Could you check a few things on this drawing? It's one solid part, dimensions in mm from its lowest x, y, z. A direction names the side the tool comes from. Give positions to 0.01 mm unless a question says otherwise; leave off trailing zeros. Loops run counter-clockwise (first coordinate to the right, second up) from the corner with the lowest first, then second, coordinate; pieces in that order, holes last. Notation, with made-up numbers: (-29.75, 31.25) -> (-2.75, 31.25) arc R7 cw to (-2.75, 39.25) -> close; hole circle Ø5 at (39, 38). An arc over 180 degrees is marked (long way). One line per question, with ' | ' between items.
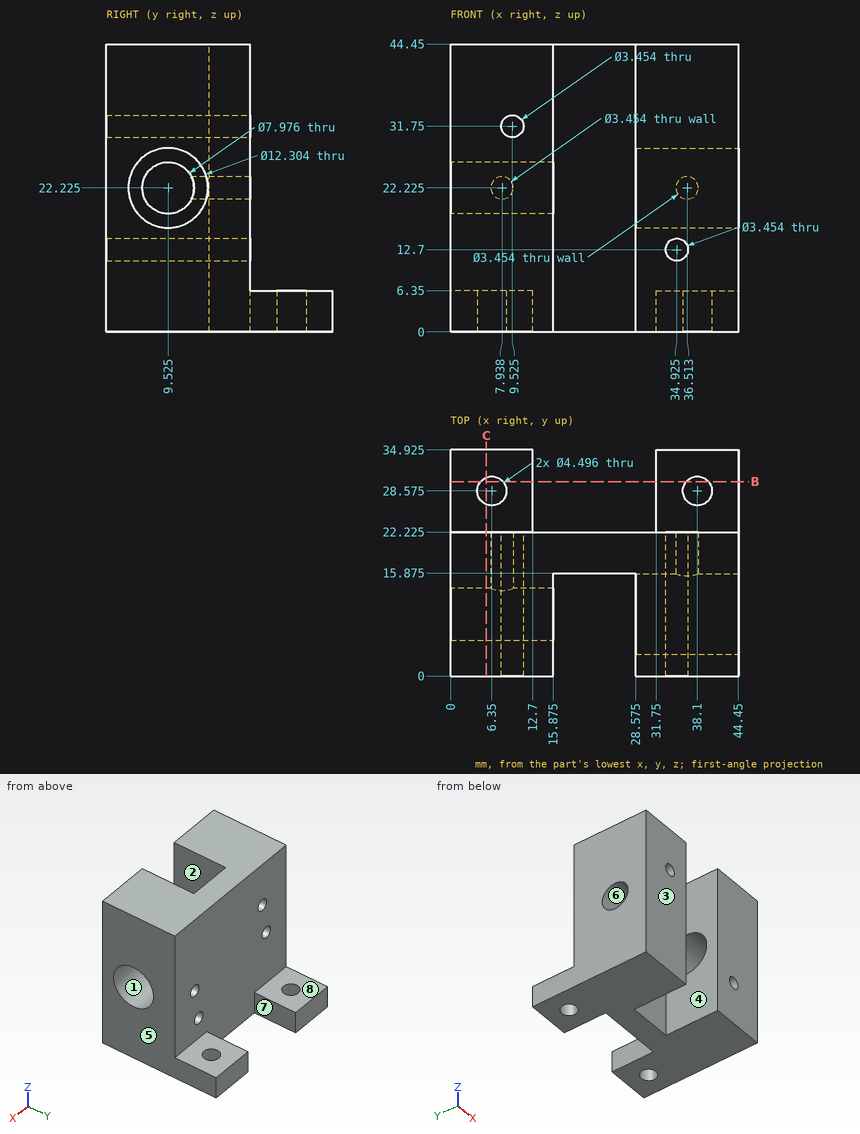
Q1. If we section it at B-B (y = 30): Write out the boundary of the cut face in (x, z).
Entries:
outline: (0, 0) -> (4.61, 0) -> (4.61, 6.35) -> (0, 6.35) -> close; (8.09, 0) -> (12.7, 0) -> (12.7, 6.35) -> (8.09, 6.35) -> close; (31.75, 0) -> (36.36, 0) -> (36.36, 6.35) -> (31.75, 6.35) -> close; (39.84, 0) -> (44.45, 0) -> (44.45, 6.35) -> (39.84, 6.35) -> close
Q2. If we mould it in two halves opening along Y, with no side actions, what happens to the marked faces 1, 2 and 3? For each: pulls with the +Y half, pulls with the -Y half, needs draft (parallel to the pull), parting line crosses it, or undercut.
Entries:
face 1: undercut | face 2: needs draft | face 3: pulls with the -Y half
Q3. If I drill on probe 1 along Y at (x, z) = (4, 41.5) (1 decimal); probe 2 along Z at (x, y) = (42, 31.5); probe 3 along Z at (x, y) = (38, 13.5), over which ranges is the centre line in solid material (lowest first)? Write a range as from..to.
Entries:
probe 1: 0..22.2 | probe 2: 0..6.35 | probe 3: 0..17.53, 26.92..44.45
Q4. For pin 1 Ø4 at (x, z) = (20.5, 6.5) entering from +Y (1 decimal); pin 2 Ø17.5 at (y, z) = (8.5, 24.5) entering from +X; pin 3 Ø5 at (x, y) = (34, 31) entering from +Z, each with a flat end and sliding along its axis, tell me the tip position at first contact or that it passes through.
Entries:
pin 1: y = 22.2 | pin 2: x = 44.45 | pin 3: z = 6.35
Q5. On a 3-axis mill with a long thin cutter (end or side, diameter ignored), from which of +Z, -Z, +X, -X, +Y, -Y can I reach the whole of each face in a straight line? I mean the marked faces 4, 5, 6, 7 and 8. Say none if no direction works.
Entries:
face 4: +Z, -Z, -Y | face 5: +Z, -Z, +X, +Y, -Y | face 6: +X, -X | face 7: +Z, -Z, +Y | face 8: +Z, +X, -X, +Y
Q6. If we section it at C-C (x = 5.5): State how many separate pieces and enclosed holes the cut face has, plus the area to 3 significant figures.
Entries:
separate pieces: 2 | enclosed holes: 1 | area: 992 mm²
